The model under review builds one solid part; all positions refer to its coordinate system, in mm. A direction names the side the tool comes from. Round coordinates to 2 decimals unless told otherwise and drop trailing zeros. Order: outer loops, then holes, each group sorted by start corner. A loop starts at its lowest first (then second) coordinate and runs counter-clockwise, first axis right, second up.
1) Mouldability with a two-part tool opening along X and no side actions: class faces 3 (the face through (-24.2, 2, -12)), 4 (the face through (0, 1, 0)), 5 (the face through (-22.6, 2, -12)) as pulls with the +X half, pulls with the -X half, needs draft (parallel to the pull), parting line crosses it, or undercut.
2) Clearance check with flat-ended pins moving along their axes: P1, Ø1.5, axis at x = 9.5, z = -12, coming from the -Y side; P2, Ø3, axis at x = 7.5, z = -10, coming from the +Y side. State where each tip first meets the part, or that it passes through.
3) Machinability: for faces 1 (the face through (0, 0, -13)), 2 (the face through (0, 1.6, -13)), which of the approach directions +Z, -Z, +X, -X, +Y, -Y give a long, thin tool a straight path to every point of the face, cutting with its end or side? Answer none if there is none.
4) Consider section C-C (x = 7.5). Give the boundary of the cut face in (y, z).
5) To check wall thickness, follow L1, parallel to X at y = 2.65, z = -8; L2, parallel to Y at x = 11.5, z = -9.5. State the ranges of each line that lie inside material, in increasing order.
6) Consider section B-B (z = -2.75). Give the boundary of the cut face in (x, y).
7) Consider section A-A (y = 2.1). Give the boundary of the cut face in (x, z), then the cut area to 3 significant figures.
from build123d import *

# Parameters (mm, degrees)
BOSS_EXTRUDE1_DEPTH = 1.6
SKETCH2_W           = 1.6
SKETCH2_H           = 25
BOSS_EXTRUDE2_DEPTH = 1.6


with BuildPart() as part:
    # Sketch1 → Boss-Extrude1 (new body)
    with BuildSketch(Plane(origin=(0, 0, 0), x_dir=(1, 0, 0), z_dir=(0, 1, 0))):
        Polygon((0, 0), (24.2, 0), (24.2, 25), (-24.2, 25), (-24.2, 0), align=None)
    extrude(amount=BOSS_EXTRUDE1_DEPTH)

    # Sketch2 → Boss-Extrude2 (add)
    with BuildSketch(Plane(origin=(0, 1.6, 0), x_dir=(1, 0, 0), z_dir=(0, 1, 0))):
        with Locations((-23.4, 12.5)):
            Rectangle(SKETCH2_W, SKETCH2_H)
        with Locations((23.4, 12.5)):
            Rectangle(SKETCH2_W, SKETCH2_H)
    extrude(amount=BOSS_EXTRUDE2_DEPTH)


solid = part.part
Answer below:
1. face 3: pulls with the -X half
1. face 4: needs draft
1. face 5: undercut
2. P1: stops at y = 0
2. P2: stops at y = 1.6
3. face 1: +Z, -Z, +X, -X, -Y
3. face 2: +Z, -Z, +Y
4. outline: (0, -25) - (1.6, -25) - (1.6, 0) - (0, 0) - close
5. L1: x = -24.2 to -22.6, 22.6 to 24.2
5. L2: y = 0 to 1.6
6. outline: (-24.2, 0) - (24.2, 0) - (24.2, 3.2) - (22.6, 3.2) - (22.6, 1.6) - (-22.6, 1.6) - (-22.6, 3.2) - (-24.2, 3.2) - close
7. outline: (-24.2, -25) - (-22.6, -25) - (-22.6, 0) - (-24.2, 0) - close; (22.6, -25) - (24.2, -25) - (24.2, 0) - (22.6, 0) - close
7. area: 80.0 mm2
